For this review, use the dimensioned drawing (mm, ordinates from the lowest corner) and the shaded views. A direction names the side the tool comes from. Coordinates: 2 decimals unless noted, no trailing zeros. Write each loop counter-clockwise with the first axis right and the second up, starting at its lowest first coordinate (ties: lowest second). Pieces come first, ordered by that corner, then holes. Notation, with made-up numbers: (76.25, -30.75) - (130.25, -30.75) arc R21 cw to (130.25, -18.75) - close; hole circle Ø1 at (77.25, 31). An arc over 180 degrees is marked (long way). One line per item, written item: value.
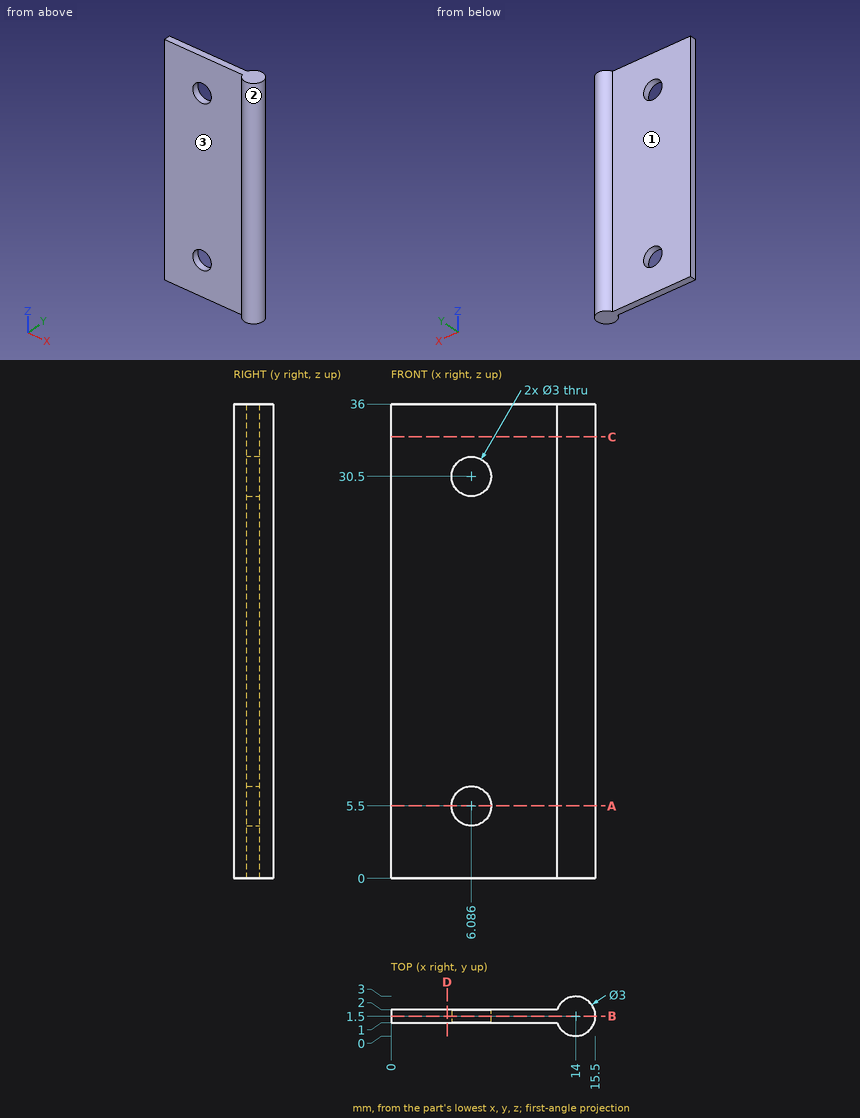
1. Consider section B-B, the plane y = 1.5. Write out the cut boundary in (x, z), then the cut area to 3 significant figures.
Answer block:
outline: (0, 0) - (15.5, 0) - (15.5, 36) - (0, 36) - close; hole circle Ø3 at (6.09, 5.5); hole circle Ø3 at (6.09, 30.5)
area: 544 mm^2
2. For the marked faces 1, 2 and 3, list the 3-axis set-ups (+Z, -Z, +X, -X, +Y, -Y) from which the entire face can be reached by the end or side of a thin tool; tool diameter is ignored.
Answer block:
face 1: +Z, -Z, -X, +Y
face 2: +Z, -Z
face 3: +Z, -Z, -X, -Y
3. Wall thickness on line 1 along Z through (x, y) = (6.75, 1.15) (1 decimal); line 2 along Y through (x, z) = (12, 15); line 3 along X through (y, z) = (1.3, 6): over which ranges is each line inside the solid? List them lowest first.
Answer block:
line 1: z = 0 to 4.2, 6.8 to 29.2, 31.8 to 36
line 2: y = 1 to 2
line 3: x = 0 to 4.67, 7.5 to 15.49
4. Consider section A-A, the plane z = 5.5. Write out the cut boundary in (x, y), then the cut area to 3 significant figures.
Answer block:
outline: (0, 1) - (4.59, 1) - (4.59, 2) - (0, 2) - close; (7.59, 1) - (12.59, 1) arc R1.5 ccw (long way) to (12.59, 2) - (7.59, 2) - close
area: 16.6 mm^2
5. Consider section D-D, the plane x = 4.25. Write out the cut boundary in (y, z), then the cut area to 3 significant figures.
Answer block:
outline: (1, 0) - (2, 0) - (2, 36) - (1, 36) - close
area: 36.0 mm^2
6. Consider section C-C, the plane z = 33.5. Write out the cut boundary in (x, y), then the cut area to 3 significant figures.
Answer block:
outline: (0, 1) - (12.59, 1) arc R1.5 ccw (long way) to (12.59, 2) - (0, 2) - close
area: 19.6 mm^2
7. Insertion check: pin 1 Ø4 at (x, z) = (6.09, 5.5) entering from -Y; pin 2 Ø6 at (x, z) = (11.5, 24.5) entering from -Y; pin 3 Ø2 at (x, z) = (3, 28.5) entering from +Y. Each pin has a flat end and moves straight along its axis. Give the tip position at first contact, or say it passes through.
Answer block:
pin 1: stops at y = 1
pin 2: stops at y = 0
pin 3: stops at y = 2
